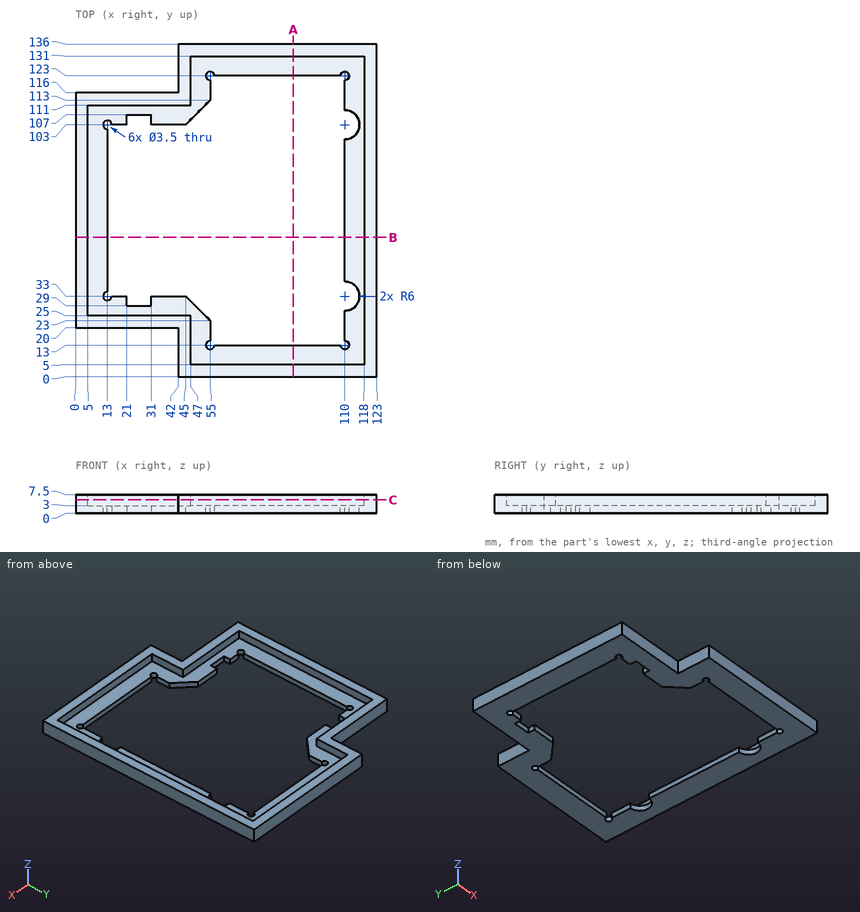
Verification items for this drawing (mm, ordinates from the low corner). Coordinates: 2 decimals unless noted, no trailing zeros. Write each loop counter-clockwise with the first axis right and the second up, starting at its lowest first coordinate (ties: lowest second). Pieces come first, ordered by that corner, then holes. Notation, with made-up numbers: M -25,41 L 34,41 A12 ccw 34,53 Z; hole C 72.5,-31 d1. An arc over 180 degrees is marked long. One line per item, written item: value. Start each with the question number.
(1) Sectioned sample at C-C, the plane z = 5.5. Enter the section's corners in (x, y).
(2) Sectioned sample at B-B, the plane y = 57. Enter the section's corners in (x, z).
(3) Sectioned sample at A-A, the plane x = 89. Enter the section's corners in (y, z).
(4) Depth check by flat-ended pin: pin 1 (4 mm diameter, centred on x = 110, y = 123, fed in from +Z); pin 2 (1.3 mm diameter, centred on x = 33.5, z = 6, fed in from -Y); pin 3 (2.5 mm diameter, centred on x = 16.5, z = 2, fed in from +Y). Enter the tip coordinate at first touch or a pass-through.
(5) Scan lines: line 1 along X through (y, z) = (121, 1.5); line 2 along Y through (x, z) = (9.5, 7.25); line 3 along X through (y, z) = (88.5, 3.5). Record each from-to range of solid material in increasing order. Write a range as [from, to].
Filled sheet:
1. outline: M 0,20 L 42,20 L 42,0 L 123,0 L 123,136 L 42,136 L 42,116 L 0,116 Z; hole M 5,25 L 47,25 L 47,5 L 118,5 L 118,131 L 47,131 L 47,111 L 5,111 Z
2. outline: M 0,0 L 13,0 L 13,3 L 5,3 L 5,7.5 L 0,7.5 Z; M 110,0 L 123,0 L 123,7.5 L 118,7.5 L 118,3 L 110,3 Z
3. outline: M 0,0 L 13,0 L 13,3 L 5,3 L 5,7.5 L 0,7.5 Z; M 123,0 L 136,0 L 136,7.5 L 131,7.5 L 131,3 L 123,3 Z
4. pin 1: z = 3
4. pin 2: y = 20
4. pin 3: y = 116
5. line 1: [42, 55], [110, 123]
5. line 2: [20, 25], [111, 116]
5. line 3: [0, 5], [118, 123]
